Verification items for the finished model (mm, model axes). A direction names the side the tool comes from. Give positions to 0.01 mm unless a question says otherwise; leave off trailing zeros. Order: outer loops, then holes, each group sorted by start corner. A loop starts at its lowest first (then second) coordinate and runs counter-clockwise, first axis right, second up.
from build123d import *

# Parameters (mm, degrees)
BASE_DEPTH                 = 25
SKETCH2_R                  = 27
SKETCH2_R_2                = 11.5
FRONT_THRU_BORDER_DEPTH    = 13
SKETCH4_R                  = 11.5
FRONT_THRU_HOLE_DEPTH      = 142.431962441
TOP_FEATURE_DEPTH          = 60
SKETCH6_R                  = 18
TOP_FEATURE_HOLE_DEPTH     = 60
SKETCH7_W                  = 90
SKETCH7_H                  = 5
TOP_FEATURE_GAP_DEPTH      = 175.38463235
SKETCH8_W                  = 20
SKETCH8_H                  = 12
TOP_FEATURE_ARM_DEPTH      = 48
FILLET2_R                  = 10
SKETCH10_R                 = 6
TOP_FEATURE_ARM_HOLE_DEPTH = 181.471604415


with BuildPart() as part:
    # Sketch1 → base (new body)
    with BuildSketch(Plane(origin=(0, 0, 0), x_dir=(1, 0, 0), z_dir=(0, 1, 0))):
        with BuildLine():
            Line((-108.1, -25.756358438), (-17.1, -54.374534481))
            ThreePointArc((-17.1, -54.374534481), (57, 0), (-17.1, 54.374534481))
            Line((-17.1, 54.374534481), (-108.1, 25.756358438))
            ThreePointArc((-108.1, 25.756358438), (-127, 0), (-108.1, -25.756358438))
        make_face()
    extrude(amount=BASE_DEPTH)

    # Sketch2 → front thru border (add)
    with BuildSketch(Plane(origin=(0, 25, 0), x_dir=(1, 0, 0), z_dir=(0, 1, 0))):
        with Locations(Location((-100, 0, 0), (0, 0, 107.457603124))):
            Circle(SKETCH2_R)
        with Locations(Location((-100, 0, 0), (0, 0, 90))):
            Circle(SKETCH2_R_2, mode=Mode.SUBTRACT)
    extrude(amount=FRONT_THRU_BORDER_DEPTH)

    # Sketch4 → front thru hole (cut, through all)
    with BuildSketch(Plane(origin=(0, 25, 0), x_dir=(1, 0, 0), z_dir=(0, 1, 0))):
        with Locations(Location((-100, 0, 0), (0, 0, 90))):
            Circle(SKETCH4_R)
    extrude(amount=-FRONT_THRU_HOLE_DEPTH, mode=Mode.SUBTRACT)

    # Sketch5 → top feature (add)
    with BuildSketch(Plane(origin=(0, 25, 0), x_dir=(1, 0, 0), z_dir=(0, 1, 0))):
        with BuildLine():
            Line((0, -27), (-40, -27))
            ThreePointArc((-40, -27), (-67, 0), (-40, 27))
            Line((-40, 27), (0, 27))
            Line((0, 27), (19, 27))
            Line((19, 27), (19, -27))
            Line((19, -27), (0, -27))
        make_face()
    extrude(amount=TOP_FEATURE_DEPTH)

    # Sketch6 → top feature hole (cut)
    with BuildSketch(Plane(origin=(0, 85, 0), x_dir=(1, 0, 0), z_dir=(0, 1, 0))):
        with Locations(Location((-40, 0, 0), (0, 0, 270))):
            Circle(SKETCH6_R)
    extrude(amount=-TOP_FEATURE_HOLE_DEPTH, mode=Mode.SUBTRACT)

    # Sketch7 → top feature gap (cut, through all)
    with BuildSketch(Plane.XY.offset(27)):
        with Locations((-26, 27.5)):
            Rectangle(SKETCH7_W, SKETCH7_H)
    extrude(amount=-TOP_FEATURE_GAP_DEPTH, mode=Mode.SUBTRACT)


with BuildPart() as top_feature_gap_piece_1:
    # of the separate pieces the step leaves, piece 1, a body of its own (top_feature_gap_pieces)
    add(part.part.solids().sort_by_distance((-17.1, 0, -54.374534481))[0])



with BuildPart() as top_feature_gap_piece_2:
    # of the separate pieces the step leaves, piece 2, a body of its own (top_feature_gap_pieces)
    add(part.part.solids().sort_by_distance((19, 30, -27))[0])


with BuildPart() as top_feature_gap_piece_1_1:
    add(top_feature_gap_piece_1.part)

    add(top_feature_gap_piece_2.part)  # top feature arm merges top feature gap piece 2
    # Sketch8 → top feature arm (add)
    with BuildSketch(Plane(origin=(0, 25, 0), x_dir=(1, 0, 0), z_dir=(0, 1, 0))):
        with Locations((0, -33)):
            Rectangle(SKETCH8_W, SKETCH8_H)
        with Locations((0, 33)):
            Rectangle(SKETCH8_W, SKETCH8_H)
    extrude(amount=TOP_FEATURE_ARM_DEPTH)

    # Fillet2
    fillet2_edges = [top_feature_gap_piece_1_1.edges().sort_by_distance(p)[0] for p in [
        (10, 73, -33),
        (-10, 73, -33),
        (10, 73, 33),
        (-10, 73, 33),
    ]]
    fillet(fillet2_edges, radius=FILLET2_R - 0.0001)  # a hair under: the kernel refuses the full size

    # Sketch10 → top feature arm hole (cut, through all)
    with BuildSketch(Plane.XY.offset(39)):
        with Locations((0, 63)):
            Circle(SKETCH10_R)
    extrude(amount=-TOP_FEATURE_ARM_HOLE_DEPTH, mode=Mode.SUBTRACT)


solid = top_feature_gap_piece_1_1.part
(1) Scan lines: line 1 (Y direction, x = 0, z = 10.5); line 2 (Z direction, x = -100, y = 34.25); line 3 (X direction, y = 11, z = 0). Record each from-to range of solid material in increasing order.
Solved:
line 1: y = 0 to 25, 30 to 57, 69 to 85
line 2: z = -27 to -11.5, 11.5 to 27
line 3: x = -127 to -111.5, -88.5 to 57
(2) Section check D-D, the plane x = -44. Enter the section's corners in (y, z), then the cut area to 3 significant figures.
Solved:
outline: (0, -45.91) - (25, -45.91) - (25, 45.91) - (0, 45.91) - close; (30, -26.7) - (85, -26.7) - (85, -17.55) - (30, -17.55) - close; (30, 17.55) - (85, 17.55) - (85, 26.7) - (30, 26.7) - close
area: 3,300 mm2
(3) Release check for a two-part mould opening along Z. For faces 6 (the flat face through (0, 27, -27)), 7 (the flat face through (-17, 57, 27)), 8 (the cylindrical face through (-4.42, 67.06, 0.55)) record: pulls with the +Z half, pulls with the -Z half, needs draft (parallel to the pull), parting line crosses it, or undercut.
Solved:
face 6: undercut
face 7: pulls with the +Z half
face 8: needs draft
(4) Go/stop test with flat-tipped pins: pin 1 (5 mm diameter, centred on y = 72.5, z = -16, fed in from -X); pin 2 (14 mm diameter, centred on x = 0, y = 63, fed in from +Z); pin 3 (1 mm diameter, centred on y = 71, z = -28.5, fed in from -X); pin 4 (8 mm diameter, centred on x = 36, y = 30, fed in from -Z). Record where each tip stops, or that it passes through.
Solved:
pin 1: stops at x = -63.38
pin 2: stops at z = 39
pin 3: stops at x = -6.61
pin 4: passes through
(5) Set-up check for faces 1 (the cylindrical face through (-7.15, 69.99, 32.92)), 2 (the flat face through (-15, 30, 0)), 3 (the flat face through (0, 49, 39)), 4 (the cylindrical face through (6.99, 70.15, 32.92)), 5 (the cylindrical face through (7.15, 69.99, -33.08)): record each of +Z, -Z, +X, -X, +Y, -Y from which the full face is reachable in a straight line by a thin tool's end or side.
Solved:
face 1: +Z, -X, +Y
face 2: +X
face 3: +Z, +X, -X, +Y
face 4: +Z, +X, +Y
face 5: -Z, +X, +Y
(6) Section check B-B, the plane z = -7. Enter the section's corners in (x, y).
Solved:
outline: (-126.08, 0) - (-109.12, 0) - (-109.12, 38) - (-126.08, 38) - close; (-90.88, 0) - (56.57, 0) - (56.57, 25) - (-73.92, 25) - (-73.92, 38) - (-90.88, 38) - close; (-66.08, 30) - (-56.58, 30) - (-56.58, 85) - (-66.08, 85) - close; (-23.42, 30) - (19, 30) - (19, 85) - (-23.42, 85) - close; hole circle Ø12 at (0, 63)
(7) Section check C-C, the plane y = 75. Enter the section's corners in (x, z), then the cut area to 3 significant figures.
Solved:
outline: (-40, -27) - (19, -27) - (19, 27) - (-40, 27) arc R27 ccw to start; hole circle Ø36 at (-40, 0)
area: 3,310 mm2
(8) Section check A-A, the plane x = -3. Enter the section's corners in (y, z), then the cut area to 3 significant figures.
Solved:
outline: (0, -56.92) - (25, -56.92) - (25, -39) - (57.8, -39) - (57.8, 39) - (25, 39) - (25, 56.92) - (0, 56.92) - close; (68.2, -39) - (72.54, -39) - (72.54, -27) - (85, -27) - (85, 27) - (72.54, 27) - (72.54, 39) - (68.2, 39) - close; hole (25, -27) - (30, -27) - (30, 27) - (25, 27) - close
area: 6,150 mm2
